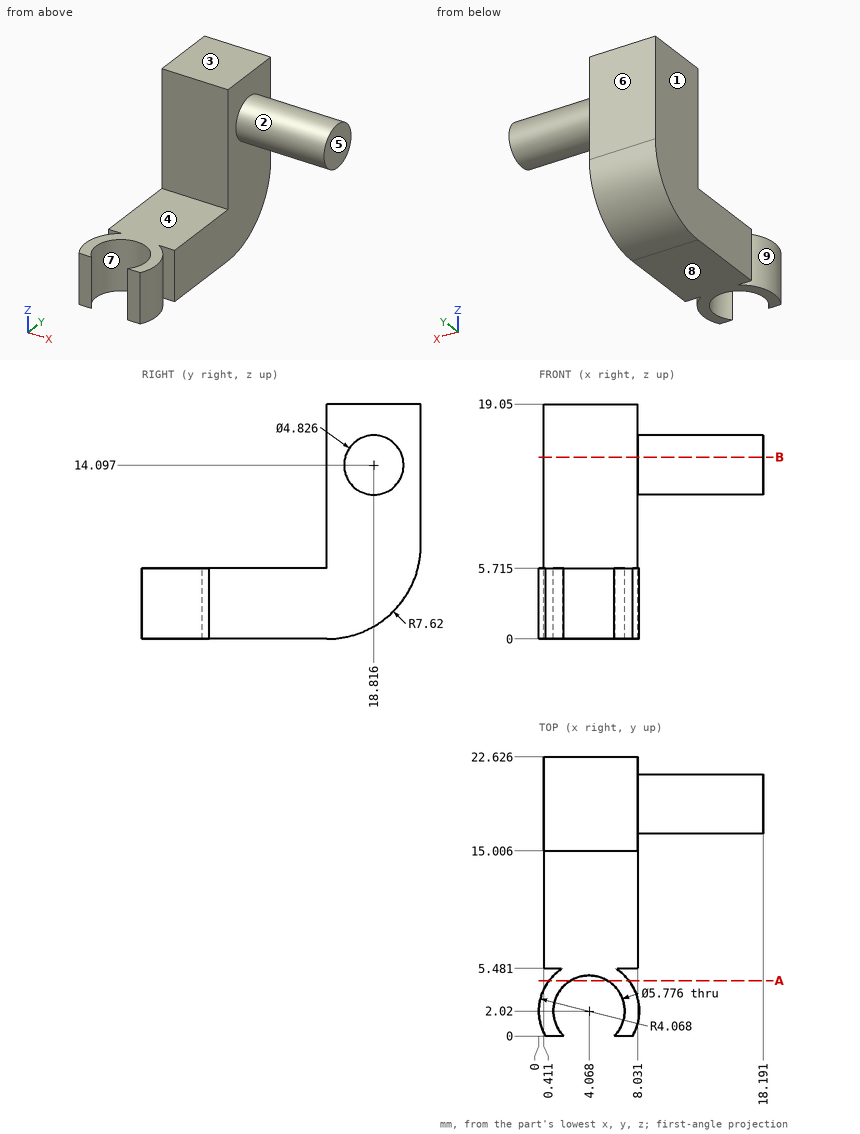
Here's the drawing with two shaded views (mm, measured from the low corner). I have some questions. A direction names the side the tool comes from. Coordinates: 2 decimals unless noted, no trailing zeros. Loops run counter-clockwise (first coordinate to the right, second up) from the corner with the lowest first, then second, coordinate; pieces in that order, holes last. Notation, with made-up numbers: M 45.25,12 L 70.25,12 A21 ccw 70.25,18 Z; hole C 20,28.25 d11. An arc over 180 degrees is marked long. Answer as CSV lines item,"result". Start each with the question number.
1. Thinking about a two-plate mould opening in Y: for the marked faces 6, 7, 8 and 9, which applies, +Y half, -Y half, draft (parallel to the pull), parting line (faces both ways), or undercut?
2. If I drill on probe 1 along X at (y, z) = (15.5, 3.5); probe 2 along Z at (x, y) = (3.25, 14.75) (1 decimal); probe 3 along Y at (x, z) = (6.5, 3.5) (1 decimal), over which ranges is the centre line in solid material (lowest first)? Write a range as [from, to].
3. For pin 1 Ø6.5 at (x, y) = (4, 6) entering from +Z (3 decimals); pin 2 Ø8.5 at (y, z) = (17.5, 13) entering from -X; pin 3 Ø5 at (x, z) = (5, 3.5) entering from -Y; pin 4 Ø5 at (x, z) = (7, 15.5) entering from -Y, each with a flat end and sliding along its axis, tell me the tip position at first contact or that it passes through.
4. For the marked faces 1, 2, 3, 4 and 5, which set-ups out of +Z, -Z, +X, -X, +Y, -Y let a thin tool reach every point of the face, with its end or its side?
5. Suppose I cut it at A-A, the plane y = 4.5. List the corners of the cut face in (x, z) for me (1 decimal).
6. Suppose I cut it at B-B, the plane z = 14.75. List the corners of the cut face in (x, y) for me (1 decimal).
Output:
1,face 6,"+Y half"
1,face 7,"undercut"
1,face 8,"draft"
1,face 9,"undercut"
2,probe 1,"x = [0.41, 8.03]"
2,probe 2,"z = [0, 5.7]"
2,probe 3,"y = [0, 0.5], [3.6, 5.3], [5.5, 21.4]"
3,pin 1,"stops at z = 5.715"
3,pin 2,"stops at x = 0.41"
3,pin 3,"stops at y = 0"
3,pin 4,"stops at y = 15.01"
4,face 1,"+Z, -Z, -X, +Y"
4,face 2,"+X"
4,face 3,"+Z, +X, -X, +Y, -Y"
4,face 4,"+Z, +X, -X, -Y"
4,face 5,"+Z, -Z, +X, +Y, -Y"
5,outline,"M 0.8,0 L 2.6,0 L 2.6,5.7 L 0.8,5.7 Z; M 5.5,0 L 7.3,0 L 7.3,5.7 L 5.5,5.7 Z"
6,outline,"M 0.4,15 L 8,15 L 8,16.5 L 18.2,16.5 L 18.2,21.1 L 8,21.1 L 8,22.6 L 0.4,22.6 Z"
